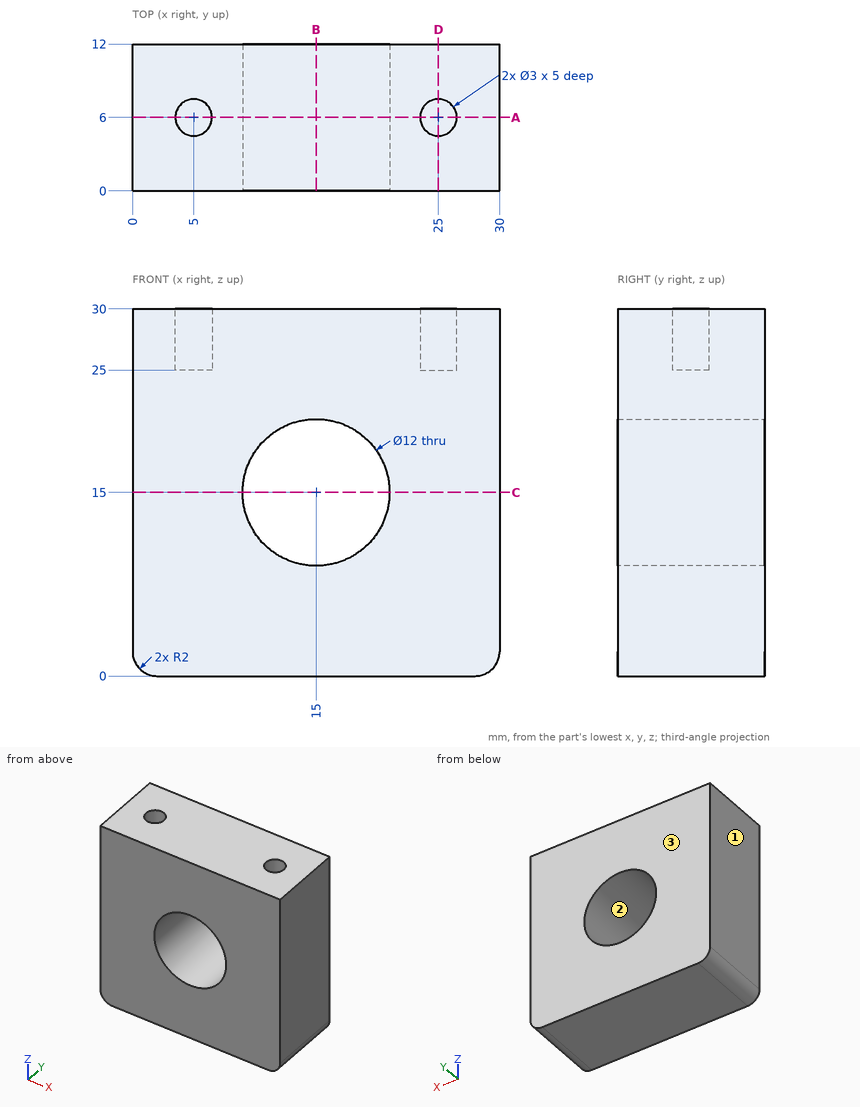
Geometry: see drawing. Coordinates: mm, zero at the bounding-box minimum. Round coordinates to 2 decimals unless told otherwise and drop trailing zeros. Loops run counter-clockwise (first coordinate to the right, second up) from the corner with the lowest first, then second, coordinate; pieces in that order, holes last. Notation, with made-up numbers: (56.5, -9.5) -> (87.5, -9.5) arc R19 cw to (87.5, 0.5) -> close; hole circle Ø7 at (80, 80.5). An arc over 180 degrees is marked (long way). One line per question, with ' | ' between items. Start each with the question number.
1. Section A-A on y = 6. Output: boundary loops of the cut face in (x, z), and give its area (3 significant figures).
2. Section D-D on x = 25. Output: boundary loops of the cut face in (y, z), and give its area (3 significant figures).
3. Section C-C on z = 15. Output: boundary loops of the cut face in (x, y).
4. Mould query, pull axis X, two halves, no side actions, for the marked faces 1, 2 and 3. Classes: pulls with the +X half, pulls with the -X half, needs draft (parallel to the pull), parting line crosses it, or undercut.
5. Section B-B on x = 15. Output: boundary loops of the cut face in (y, z).
6. Contact query for flat-ended pins moving along their axis: pin 1 (11 mm diameter, centred on x = 15, z = 15, fed in from -Y); pin 2 (1.5 mm diameter, centred on x = 25, y = 5.5, fed in from +Z). Output: stop coordinate, or through.
7. Line query: line 1 along X through (y, z) = (9, 15); line 2 along Z through (x, y) = (17, 7.5); line 3 along Z through (x, y) = (17.25, 5). Output: solid intervals per line, ascending. Write a range as [from, to].
Returned:
1) outline: (0, 2) arc R2 ccw to (2, 0) -> (28, 0) arc R2 ccw to (30, 2) -> (30, 30) -> (26.5, 30) -> (26.5, 25) -> (23.5, 25) -> (23.5, 30) -> (6.5, 30) -> (6.5, 25) -> (3.5, 25) -> (3.5, 30) -> (0, 30) -> close; hole circle Ø12 at (15, 15) | area: 755 mm2
2) outline: (0, 0) -> (12, 0) -> (12, 30) -> (7.5, 30) -> (7.5, 25) -> (4.5, 25) -> (4.5, 30) -> (0, 30) -> close | area: 345 mm2
3) outline: (0, 0) -> (9, 0) -> (9, 12) -> (0, 12) -> close; (21, 0) -> (30, 0) -> (30, 12) -> (21, 12) -> close
4) face 1: pulls with the -X half | face 2: undercut | face 3: needs draft
5) outline: (0, 0) -> (12, 0) -> (12, 9) -> (0, 9) -> close; (0, 21) -> (12, 21) -> (12, 30) -> (0, 30) -> close
6) pin 1: passes through | pin 2: stops at z = 25
7) line 1: x = [0, 9], [21, 30] | line 2: z = [0, 9.34], [20.66, 30] | line 3: z = [0, 9.44], [20.56, 30]
